For this review, take the finished solid that the model builds, in its own axes (mm). A direction names the side the tool comes from. Coordinates: 2 decimals unless noted, no trailing zeros. Loops run counter-clockwise (first coordinate to the right, second up) from the corner with the lowest first, then second, coordinate; pieces in that order, holes last. Notation, with made-up numbers: M 32,26.5 L 65,26.5 A23 ccw 65,50.5 Z; hole C 30.5,-38.75 d10. An arc over 180 degrees is marked long. Answer as a JSON object with one key per item and string values. Group by question number.
Item 1: Insertion check: pin 1 (4 mm diameter, centred on x = -50.5, z = 0.5, fed in from -Y) (3 decimals); pin 2 (0.7 mm diameter, centred on x = -51, z = 11, fed in from -Y); pin 3 (6 mm diameter, centred on x = -40.5, z = -1, fed in from +Y); pin 4 (8.5 mm diameter, centred on x = 0, z = 0, fed in from -Y). Each pin has a flat end and moves straight along its axis. Give the tip position at first contact, or say it passes through.
Item 2: Add section C-C (x = -27). State the section outline as (y, z) points.
Item 3: Add section A-A (y = 0). State the section outline as (x, z) points (1 decimal).
Item 4: Wall thickness on L1, parallel to Y at x = -10, z = 6; L2, parallel to Z at x = -51.5, y = 0.5; L3, parallel to Y at x = -23.5, z = -18.5: over which ranges is each line inside the solid? List them lowest first. Write a range as from..to.
Item 5: Add section D-D (y = 22.5). State the section outline as (x, z) points.
Item 6: Tool access review of faces 1 (the face through (-51, -9.525, 0)), 2 (the face through (-8, 26.988, 0)), 3 (the face through (-52, -22.225, 3)), 4 (the face through (-48, -2.381, 10)), 5 (the face through (-51, -18.923, 0)): name each direction out of +Z, -Z, +X, -X, +Y, -Y from which nothing blocks a thin tool from reaching the whole face with its end or side.
Item 7: Add section B-B (x = -13). State the section outline as (y, z) points.
Item 8: Mouldability with a two-part tool opening along X and no side actions: class faces 6 (the face through (-8.99, 29.34, -15.43)), 7 (the face through (-8, -26.988, 0)), 8 (the face through (-52.603, -20.597, -2.053)) as +X half, -X half, draft (parallel to the pull), parting line (faces both ways), or undercut.
from build123d import *

# Parameters (mm, degrees)
SKETCH1_W           = 30.559375
SKETCH1_H           = 20.6375
BOSS_EXTRUDE6_DEPTH = 31.75
CHAMFER1_SIZE       = 2.06375
EXTRUDE3_DEPTH      = 75.228527622
EXTRUDE3_DEPTH_BACK = 75.228527622
EXTRUDE1_DEPTH      = 75.228527622
EXTRUDE1_DEPTH_BACK = 75.228527622
SKETCH4_R           = 9.525
EXTRUDE4_DEPTH      = 30.559375
EXTRUDE6_DEPTH      = 75.228527694
EXTRUDE6_DEPTH_BACK = 75.228527694
SKETCH6_R           = 7.14375
SKETCH33_W          = 2.38125
SKETCH33_H          = 4.7625
CUT_EXTRUDE1_DEPTH  = 87.767041438
SKETCH34_R          = 4.7625
CUT_EXTRUDE2_DEPTH  = 75.228527694
CUT_EXTRUDE3_DEPTH  = 3.302


with BuildPart() as part:
    # Sketch1 → Revolve1 (revolve)
    with BuildSketch(Plane(origin=(0, 0, 0), x_dir=(1, 0, 0), z_dir=(0, 1, 0)), mode=Mode.PRIVATE) as revolve1_sk:
        with Locations((-48.2203125, 10.31875)):
            Rectangle(SKETCH1_W, SKETCH1_H)
    revolve(revolve1_sk.sketch.rotate(Axis((-63.5, 0, 0), (1, 0, 0)), 180), axis=Axis((-63.5, 0, 0), (1, 0, 0)))

    # Sketch30 → Boss-Extrude6 (add, symmetric)
    with BuildSketch(Plane(origin=(0, 0, 0), x_dir=(1, 0, 0), z_dir=(0, 1, 0))):
        Polygon((-39.290625, 21.669375), (-39.290625, -21.669375), (-21.828125, -21.669375), (14.2875, -21.669375), (14.2875, 21.669375), (-21.828125, 21.669375), align=None)
    extrude(amount=BOSS_EXTRUDE6_DEPTH, both=True)

    # Chamfer1
    chamfer1_edges = [part.edges().sort_by_distance(p)[0] for p in [
        (-63.5, 0, -20.6375),
    ]]
    chamfer(chamfer1_edges, length=CHAMFER1_SIZE)

    # Sketch3 → Extrude3 (cut, two sides: drawn at the far end of the back side and taken through both)
    with BuildSketch(Plane.XY.offset(-EXTRUDE3_DEPTH_BACK)):
        with BuildLine():
            Line((-21.828125, 26.9875), (32.940625, 26.9875))
            Line((32.940625, 26.9875), (32.940625, -26.9875))
            Line((32.940625, -26.9875), (-21.828125, -26.9875))
            ThreePointArc((-21.828125, -26.9875), (-29.685849106, -23.732724106), (-32.940625, -15.875))
            Line((-32.940625, -15.875), (-32.940625, 15.875))
            ThreePointArc((-32.940625, 15.875), (-29.685849106, 23.732724106), (-21.828125, 26.9875))
        make_face()
        with BuildLine():
            Line((-39.290625, 31.75), (-28.178125, 31.75))
            ThreePointArc((-28.178125, 31.75), (-36.035849106, 28.495224106), (-39.290625, 20.6375))
            Line((-39.290625, 20.6375), (-39.290625, 31.75))
        make_face()
        with BuildLine():
            Line((-39.290625, -31.75), (-39.290625, -20.6375))
            ThreePointArc((-39.290625, -20.6375), (-36.035849106, -28.495224106), (-28.178125, -31.75))
            Line((-28.178125, -31.75), (-39.290625, -31.75))
        make_face()
    extrude(amount=EXTRUDE3_DEPTH + EXTRUDE3_DEPTH_BACK, mode=Mode.SUBTRACT)

    # Sketch2 → Extrude1 (cut, two sides: drawn at the far end of the back side and taken through both)
    with BuildSketch(Plane(origin=(0, 0, 0), x_dir=(1, 0, 0), z_dir=(0, 1, 0)).offset(-EXTRUDE1_DEPTH_BACK)):
        with BuildLine():
            Line((20.6375, 31.75), (20.6375, -31.75))
            Line((20.6375, -31.75), (-21.828125, -31.75))
            Line((-21.828125, -31.75), (-28.178125, -21.669375))
            ThreePointArc((-28.178125, -21.669375), (-22.727549003, -20.967272623), (-17.632826724, -18.906803902))
            ThreePointArc((-17.632826724, -18.906803902), (-9.113925428, -15.461487614), (0, -14.2875))
            ThreePointArc((0, -14.2875), (14.2875, 0), (0, 14.2875))
            ThreePointArc((0, 14.2875), (-9.113925428, 15.461487614), (-17.632826724, 18.906803902))
            ThreePointArc((-17.632826724, 18.906803902), (-22.727549003, 20.967272623), (-28.178125, 21.669375))
            Line((-28.178125, 21.669375), (-21.828125, 31.75))
            Line((-21.828125, 31.75), (20.6375, 31.75))
        make_face()
    extrude(amount=EXTRUDE1_DEPTH + EXTRUDE1_DEPTH_BACK, mode=Mode.SUBTRACT)

    # Sketch4 → Extrude4 (cut)
    with BuildSketch(Plane.ZY.offset(63.5)):
        Circle(SKETCH4_R)
    extrude(amount=-EXTRUDE4_DEPTH, mode=Mode.SUBTRACT)

    # Sketch6 → Extrude6 (cut, two sides: drawn at the far end of the back side and taken through both)
    with BuildSketch(Plane(origin=(0, 0, 0), x_dir=(1, 0, 0), z_dir=(0, 1, 0)).offset(-EXTRUDE6_DEPTH_BACK)):
        with Locations(Location((0, 0, 0), (0, 0, 270))):
            Circle(SKETCH6_R)
    extrude(amount=EXTRUDE6_DEPTH + EXTRUDE6_DEPTH_BACK, mode=Mode.SUBTRACT)

    # Sketch33 → Cut-Extrude1 (cut, through all)
    with BuildSketch(Plane.ZY.offset(63.5)):
        with Locations((10.413166593, 0)):
            Rectangle(SKETCH33_W, SKETCH33_H)
    extrude(amount=-CUT_EXTRUDE1_DEPTH, mode=Mode.SUBTRACT)

    # Sketch34 → Cut-Extrude2 (cut, through all)
    with BuildSketch(Plane(origin=(0, 0, 0), x_dir=(1, 0, 0), z_dir=(0, 1, 0))):
        with Locations(Location((-51.3953125, 0, 0), (0, 0, 270))):
            Circle(SKETCH34_R)
    extrude(amount=-CUT_EXTRUDE2_DEPTH, mode=Mode.SUBTRACT)

    # Sketch35 → Revolve2 (revolve)
    with BuildSketch(Plane(origin=(-51.3953125, 0, 0), x_dir=(0, 0, -1), z_dir=(1, 0, 0))):
        Polygon((-3.96875, -9.525), (-4.7625, -10.31875), (-4.7625, -21.43125), (-3.96875, -22.225), (0, -22.225), (0, -9.525), align=None)
    revolve(axis=Axis((-51.3953125, -9.525, 0), (0, -1, 0)))

    # Sketch36 → Cut-Extrude3 (cut)
    with BuildSketch(Plane.XZ.offset(22.225)):
        Polygon((-51.3953125, -2.749630657), (-49.0140625, -1.374815329), (-49.0140625, 1.374815329), (-51.3953125, 2.749630657), (-53.7765625, 1.374815329), (-53.7765625, -1.374815329), align=None)
    extrude(amount=-CUT_EXTRUDE3_DEPTH, mode=Mode.SUBTRACT)

    # Cut-Extrude4 cone 1 section (through the dimple's axis) → Cut-Extrude4 (revolve, cut)
    with BuildSketch(Plane(origin=(-51.3953125, -22.225, 0), x_dir=(0, 0, -1), z_dir=(1, 0, 0))):
        Polygon((0, 0), (2.749630657, 0), (0, 2.749630657), align=None)
    revolve(axis=Axis((-51.3953125, -22.225, 0), (0, 1, 0)), mode=Mode.SUBTRACT)


solid = part.part
From the geometry:
{
 "1": {"pin 1": "stops at y = -22.225", "pin 2": "stops at y = -17.68", "pin 3": "stops at y = 26.69", "pin 4": "passes through"},
 "2": {"outline": "M -31.75,-21.64 L -25.71,-21.64 L -25.71,21.64 L -31.75,21.64 Z; M 25.71,-21.64 L 31.75,-21.64 L 31.75,21.64 L 25.71,21.64 Z"},
 "3": {"outline": "M -63.5,-18.6 L -61.4,-20.6 L -39.3,-20.6 L -39.3,-21.7 L -32.9,-21.7 L -32.9,-9.5 L -63.5,-9.5 Z; M -63.5,11.6 L -32.9,11.6 L -32.9,21.7 L -39.3,21.7 L -39.3,20.6 L -61.4,20.6 L -63.5,18.6 Z"},
 "4": {"L1": "y = -31.75..-26.99, 26.99..31.75", "L2": "z = -20.63..-9.51, 11.6..20.63", "L3": "y = -31.75..-26.86, 26.86..31.75"},
 "5": {"outline": "M -39.13,-21.67 L -30.75,-21.67 L -30.75,21.67 L -39.13,21.67 Z"},
 "6": {"face 1": "none", "face 2": "+Z, -Z, +X", "face 3": "+Z, -Z, -X, -Y", "face 4": "+X, -X", "face 5": "-Y"},
 "7": {"outline": "M -31.75,-16.72 L -26.99,-16.72 L -26.99,16.72 L -31.75,16.72 Z; M 26.99,-16.72 L 31.75,-16.72 L 31.75,16.72 L 26.99,16.72 Z"},
 "8": {"face 6": "+X half", "face 7": "draft", "face 8": "undercut"}
}
